For this review, take the finished solid that the model builds, in its own axes (mm). A direction names the side the tool comes from. Coordinates: 2 decimals unless noted, no trailing zeros. Loops run counter-clockwise (first coordinate to the right, second up) from the corner with the lowest first, then second, coordinate; pieces in that order, holes last. Notation, with made-up numbers: M 20,65.25 L 69,65.25 A26 cw 69,103.25 Z; hole C 66,75 d7. An arc over 180 degrees is marked long. Answer as a JSON object with one key per item and string values. Group by question number.
Item 1: Mouldability with a two-part tool opening along Z and no side actions: class faces 1 (the face through (-219, 3, -53.064)), 2 (the face through (-153, 3, -84.471)), 3 (the face through (-147, 6.35, -17)) as +Z half, -Z half, draft (parallel to the pull), parting line (faces both ways), or undercut.
Item 2: Add section B-B (z = 42). State the section outline as (x, y) points, then the cut area to 3 significant figures.
Item 3: Add section A-A (z = -38). State the section outline as (x, y) points.
Item 4: Add section C-C (y = 5). Count the separate pieces of the cut face and the enclosed holes in it, then the cut area to 3 significant figures.
Item 5: Tool access review of faces 4 (the face through (-237, 3, -54.626)), 5 (the face through (-189.821, 3, -37)), 6 (the face through (-62.515, 3, 3)): name each direction out of +Z, -Z, +X, -X, +Y, -Y from which nothing blocks a thin tool from reaching the whole face with its end or side.
Item 6: Add section D-D (z = -61). State the section outline as (x, y) points.
Item 7: Insertion check: pin 1 (1.9 mm diameter, centred on x = -237.16, z = -41.93, fed in from -Y); pin 2 (0.5 mm diameter, centred on y = 3.5, z = -19, fed in from -X); pin 3 (2 mm diameter, centred on x = -66.5, y = 2, fed in from -Z); pin 4 (0.9 mm diameter, centred on y = 4.5, z = -31.5, fed in from +X). Each pin has a flat end and moves straight along its axis. Give the tip position at first contact, or say it passes through.
Item 8: Wall thickness on L1, parallel to Z at x = -192, y = 1.75; L2, parallel to X at y = 4, z = 31.5; L3, parallel to Z at x = -186, y = 6.25: over which ranges is each line inside the solid? List them lowest first. Write a range as from..to.
from build123d import *

# Parameters (mm, degrees)
SKETCH1_R           = 1.5875
SKETCH1_W           = 6.096
SKETCH1_H           = 6.35
BOSS_EXTRUDE1_DEPTH = 6.35


with BuildPart() as part:
    # Sketch1 → Boss-Extrude1 (new body)
    with BuildSketch(Plane(origin=(0, 0, 0), x_dir=(1, 0, 0), z_dir=(0, 1, 0))):
        with BuildLine():
            Line((-233.985969077, 84.470905347), (-68.885969077, 84.470905347))
            ThreePointArc((-68.885969077, 84.470905347), (-59.905712956, 80.751161468), (-56.185969077, 71.770905347))
            Line((-56.185969077, 71.770905347), (-56.174553175, 41.925905347))
            Line((-56.174553175, 41.925905347), (-62.514837513, 41.925905347))
            Line((-62.514837513, 41.925905347), (-62.514837513, 30.749799864))
            Line((-62.514837513, 30.749799864), (-65.689837513, 30.749799864))
            Line((-65.689837513, 30.749799864), (-65.689837513, 32.502399864))
            Line((-65.689837513, 32.502399864), (-68.229837513, 32.502399864))
            Line((-68.229837513, 32.502399864), (-68.229837513, 30.749799864))
            Line((-68.229837513, 30.749799864), (-69.499837513, 30.749799864))
            Line((-69.499837513, 30.749799864), (-69.499837513, 27.701940508))
            Line((-69.499837513, 27.701940508), (-68.229837513, 27.701940508))
            Line((-68.229837513, 27.701940508), (-68.229837513, 25.949340508))
            Line((-68.229837513, 25.949340508), (-65.689837513, 25.949340508))
            Line((-65.689837513, 25.949340508), (-65.689837513, 27.701940508))
            Line((-65.689837513, 27.701940508), (-62.514837513, 27.701940508))
            Line((-62.514837513, 27.701940508), (-62.514837513, 16.525905347))
            Line((-62.514837513, 16.525905347), (-62.514837513, 5.349799864))
            Line((-62.514837513, 5.349799864), (-65.689837513, 5.349799864))
            Line((-65.689837513, 5.349799864), (-65.689837513, 7.102399864))
            Line((-65.689837513, 7.102399864), (-68.229837513, 7.102399864))
            Line((-68.229837513, 7.102399864), (-68.229837513, 5.349799864))
            Line((-68.229837513, 5.349799864), (-69.499837513, 5.349799864))
            Line((-69.499837513, 5.349799864), (-69.499837513, 2.301940508))
            Line((-69.499837513, 2.301940508), (-68.229837513, 2.301940508))
            Line((-68.229837513, 2.301940508), (-68.229837513, 0.549340508))
            Line((-68.229837513, 0.549340508), (-65.689837513, 0.549340508))
            Line((-65.689837513, 0.549340508), (-65.689837513, 2.301940508))
            Line((-65.689837513, 2.301940508), (-62.514837513, 2.301940508))
            Line((-62.514837513, 2.301940508), (-62.514837513, -8.874094653))
            Line((-62.514837513, -8.874094653), (-56.155121852, -8.874094653))
            Line((-56.155121852, -8.874094653), (-56.14370595, -38.719094653))
            ThreePointArc((-56.14370595, -38.719094653), (-59.863449829, -47.699350774), (-68.84370595, -51.419094653))
            Line((-68.84370595, -51.419094653), (-233.985969077, -51.419094653))
            Line((-233.985969077, -51.419094653), (-233.985969077, -45.069094653))
            Line((-233.985969077, -45.069094653), (-233.985969077, -35.798024331))
            Line((-233.985969077, -35.798024331), (-230.810969077, -35.798024331))
            Line((-230.810969077, -35.798024331), (-230.810969077, -37.550624331))
            Line((-230.810969077, -37.550624331), (-228.270969077, -37.550624331))
            Line((-228.270969077, -37.550624331), (-228.270969077, -35.798024331))
            Line((-228.270969077, -35.798024331), (-227.000969077, -35.798024331))
            Line((-227.000969077, -35.798024331), (-227.000969077, -32.750164975))
            Line((-227.000969077, -32.750164975), (-228.270969077, -32.750164975))
            Line((-228.270969077, -32.750164975), (-228.270969077, -30.997564975))
            Line((-228.270969077, -30.997564975), (-230.810969077, -30.997564975))
            Line((-230.810969077, -30.997564975), (-230.810969077, -32.750164975))
            Line((-230.810969077, -32.750164975), (-233.985969077, -32.750164975))
            Line((-233.985969077, -32.750164975), (-233.985969077, -21.574094653))
            Line((-233.985969077, -21.574094653), (-240.335969077, -21.574094653))
            Line((-240.335969077, -21.574094653), (-240.335969077, 3.825905347))
            Line((-240.335969077, 3.825905347), (-233.985969077, 3.825905347))
            Line((-233.985969077, 3.825905347), (-233.985969077, 15.001975669))
            Line((-233.985969077, 15.001975669), (-230.810969077, 15.001975669))
            Line((-230.810969077, 15.001975669), (-230.810969077, 13.249375669))
            Line((-230.810969077, 13.249375669), (-228.270969077, 13.249375669))
            Line((-228.270969077, 13.249375669), (-228.270969077, 15.001975669))
            Line((-228.270969077, 15.001975669), (-227.000969077, 15.001975669))
            Line((-227.000969077, 15.001975669), (-227.000969077, 18.049835025))
            Line((-227.000969077, 18.049835025), (-228.270969077, 18.049835025))
            Line((-228.270969077, 18.049835025), (-228.270969077, 19.802435025))
            Line((-228.270969077, 19.802435025), (-230.810969077, 19.802435025))
            Line((-230.810969077, 19.802435025), (-230.810969077, 18.049835025))
            Line((-230.810969077, 18.049835025), (-233.985969077, 18.049835025))
            Line((-233.985969077, 18.049835025), (-233.985969077, 29.225905347))
            Line((-233.985969077, 29.225905347), (-240.335969077, 29.225905347))
            Line((-240.335969077, 29.225905347), (-240.335969077, 54.625905347))
            Line((-240.335969077, 54.625905347), (-233.985969077, 54.625905347))
            Line((-233.985969077, 54.625905347), (-233.985969077, 65.801975669))
            Line((-233.985969077, 65.801975669), (-230.810969077, 65.801975669))
            Line((-230.810969077, 65.801975669), (-230.810969077, 64.049375669))
            Line((-230.810969077, 64.049375669), (-228.270969077, 64.049375669))
            Line((-228.270969077, 64.049375669), (-228.270969077, 65.801975669))
            Line((-228.270969077, 65.801975669), (-227.000969077, 65.801975669))
            Line((-227.000969077, 65.801975669), (-227.000969077, 68.849835025))
            Line((-227.000969077, 68.849835025), (-228.270969077, 68.849835025))
            Line((-228.270969077, 68.849835025), (-228.270969077, 70.602435025))
            Line((-228.270969077, 70.602435025), (-230.810969077, 70.602435025))
            Line((-230.810969077, 70.602435025), (-230.810969077, 68.849835025))
            Line((-230.810969077, 68.849835025), (-233.985969077, 68.849835025))
            Line((-233.985969077, 68.849835025), (-233.985969077, 78.120905347))
            Line((-233.985969077, 78.120905347), (-233.985969077, 84.470905347))
        make_face()
        with Locations(Location((-237.160969077, 41.925905347, 0), (0, 0, 270))):
            Circle(SKETCH1_R, mode=Mode.SUBTRACT)
        with Locations(Location((-237.160969077, -8.874094653, 0), (0, 0, 270))):
            Circle(SKETCH1_R, mode=Mode.SUBTRACT)
        with Locations(Location((-186.646041016, 16.54252462, 0), (0, 0, 270))):
            Circle(SKETCH1_R, mode=Mode.SUBTRACT)
        with Locations(Location((-205.696041016, -16.836994653, 0), (0, 0, 270))):
            Circle(SKETCH1_R, mode=Mode.SUBTRACT)
        with Locations(Location((-205.696041016, 49.888805347, 0), (0, 0, 270))):
            Circle(SKETCH1_R, mode=Mode.SUBTRACT)
        Polygon((-189.821041016, -20.011994653), (-183.471041016, -20.011994653), (-183.471041016, 5.388005347), (-189.821041016, 5.388005347), (-189.821041016, -13.661994653), (-195.917041016, -13.661994653), (-195.917041016, -20.011994653), align=None, mode=Mode.SUBTRACT)
        Polygon((-189.821041016, 53.063805347), (-183.471041016, 53.063805347), (-183.471041016, 27.663805347), (-189.821041016, 27.663805347), (-189.821041016, 46.713805347), (-195.917041016, 46.713805347), (-195.917041016, 53.063805347), align=None, mode=Mode.SUBTRACT)
        with Locations((-218.523041016, -16.836994653)):
            Rectangle(SKETCH1_W, SKETCH1_H, mode=Mode.SUBTRACT)
        with Locations((-218.523041016, 49.888805347)):
            Rectangle(SKETCH1_W, SKETCH1_H, mode=Mode.SUBTRACT)
    extrude(amount=BOSS_EXTRUDE1_DEPTH)


solid = part.part
From the geometry:
{
 "1": {"face 1": "undercut", "face 2": "-Z half", "face 3": "draft"},
 "2": {"outline": "M -233.99,0 L -56.57,0 L -56.57,6.35 L -233.99,6.35 Z", "area": "1,130 mm²"},
 "3": {"outline": "M -240.34,0 L -189.82,0 L -189.82,6.35 L -240.34,6.35 Z; M -183.47,0 L -62.51,0 L -62.51,6.35 L -183.47,6.35 Z"},
 "4": {"separate pieces": "1", "enclosed holes": "9", "area": "23,400 mm²"},
 "5": {"face 4": "-Z, -X, +Y, -Y", "face 5": "+Y, -Y", "face 6": "+X, +Y, -Y"},
 "6": {"outline": "M -233.99,0 L -56.18,0 L -56.18,6.35 L -233.99,6.35 Z"},
 "7": {"pin 1": "passes through", "pin 2": "stops at x = -233.99", "pin 3": "stops at z = -84.4", "pin 4": "stops at x = -62.51"},
 "8": {"L1": "z = -84.47..-53.06, -46.71..13.66, 20.01..51.42", "L2": "x = -233.99..-230.81, -228.27..-56.15", "L3": "z = -84.47..-53.06, -27.66..-17.99, -15.09..-5.39, 20.01..51.42"}
}
